Check sheet for the modelled part. Datum: model origin and axes. Units: mm. A direction names the side the tool comes from. Coordinates: 2 decimals unless noted, no trailing zeros. Write each loop counter-clockwise with the first axis right and the second up, starting at its lowest first coordinate (ties: lowest second). Pieces come first, ordered by that corner, then holes. Notation, with made-up numbers: (-31.5, 13.5) - (21.5, 13.5) arc R32 cw to (21.5, 50.5) - close; hole circle Ø9 at (18.25, 72.25). An arc over 180 degrees is marked (long way). Use one line per item in the form item = value. Start each with the question number.
1. Tool access check on faces 1 (the face through (-10, -10, 5)), 2 (the face through (34.997, -21, 15)). Record the directions out of +Z, -Z, +X, -X, +Y, -Y that give a thin tool (end or side, any length) a straight path to the whole face; none if there is none.
2. Cross-section at C-C on y = 8. Record the boundary of the cut face in (x, z), then the cut area to 3 significant figures.
3. Go/stop test with flat-tipped pins: pin 1 Ø1.5 at (x, y) = (-25.5, 10) entering from -Z; pin 2 Ø3.5 at (x, y) = (-15.5, -15.5) entering from +Z; pin 3 Ø5.5 at (x, z) = (30.23, 4.76) entering from +Y; pin 4 Ø1.8 at (x, y) = (15.5, 15.5) entering from -Z. Record where each tip stops, or that it passes through.
4. Scan lines: line 1 along Y through (x, z) = (0, 3); line 2 along X through (y, z) = (6, 15.5); line 3 along Z through (x, y) = (-18.5, 19). Record each from-to range of solid material in increasing order.
5. Cross-section at A-A on x = 0. Record the boundary of the cut face in (y, z), then the cut area to 3 significant figures.
6. Cross-section at D-D on x = 30.5. Record the boundary of the cut face in (y, z), then the cut area to 3 significant figures.
7. Cross-section at B-B on z = 16.5. Record the boundary of the cut face in (x, y), then the cut area to 3 significant figures.
8. Draft check along Z on faces 3 (the face through (-23.86, 1.71, 18.66)), 4 (the face through (30, -19.122, 15)), 5 (the face through (32.385, -20.687, 4.857)), 6 (the face through (-28.084, -20.687, 4.857)). Enter one of: +Z half, -Z half, draft (parallel to the pull), parting line (faces both ways), or undercut.
```python
from build123d import *

# Parameters (mm, degrees)
F0_R     = 1.5
F0_R_2   = 11.253
F1_DEPTH = 5
F3_DEPTH = 25.4
F4_R     = 2.15265
F5_DEPTH = 3.175
F7_DEPTH = 50.943485


with BuildPart() as f1:
    # F0 (on Top) → F1 (new body)
    with BuildSketch(Plane.XY):
        Polygon((25.471742, 21.502992), (-25.471742, 21.502992), (-25.471742, -19.121742), (-34.996742, -19.121742), (-34.996742, -22.296742), (34.996742, -22.296742), (34.996742, -19.121742), (25.471742, -19.121742), align=None)
        with Locations((-15.499994, -15.499994)):
            Circle(F0_R, mode=Mode.SUBTRACT)
        with Locations((15.499994, -15.499994)):
            Circle(F0_R, mode=Mode.SUBTRACT)
        Circle(F0_R_2, mode=Mode.SUBTRACT)
        with Locations((-15.499994, 15.499994)):
            Circle(F0_R, mode=Mode.SUBTRACT)
        with Locations((15.499994, 15.499994)):
            Circle(F0_R, mode=Mode.SUBTRACT)
    extrude(amount=F1_DEPTH)

    # F2 (on face) → F3 (join)
    with BuildSketch(Plane.XY.offset(5)):
        Polygon((-34.996742, -19.121742), (-34.996742, -22.296742), (-22.296742, -22.296742), (-22.296742, 21.502992), (-25.471742, 21.502992), (-25.471742, -19.121742), align=None)
        Polygon((25.471742, -19.121742), (25.471742, 21.502992), (22.296742, 21.502992), (22.296742, -22.296742), (34.996742, -22.296742), (34.996742, -19.121742), align=None)
    extrude(amount=F3_DEPTH)

    # F4 (on face) → F5 (cut, through all)
    with BuildSketch(Plane(origin=(0, -19.121742, 0), x_dir=(-1, 0, 0), z_dir=(0, 1, 0))):
        with Locations((30.234242, 4.7625)):
            Circle(F4_R)
        with Locations((30.234242, 25.6375)):
            Circle(F4_R)
        with Locations((-30.234242, 25.6375)):
            Circle(F4_R)
        with Locations((-30.234242, 4.7625)):
            Circle(F4_R)
    extrude(amount=-F5_DEPTH, mode=Mode.SUBTRACT)

    # F6 (on face) → F7 (cut, through all)
    with BuildSketch(Plane.YZ.offset(25.471742)):
        Polygon((21.502992, 6.5875), (21.502992, 30.4), (-17.534242, 30.4), align=None)
    extrude(amount=-F7_DEPTH, mode=Mode.SUBTRACT)


solid = f1.part
```
Final values:
q1.face_1 = +Z, +Y, -Y
q1.face_2 = +Z, -Z, +X, +Y, -Y
q2.outline = (-25.47, 0) - (-7.91, 0) - (-7.91, 5) - (-22.3, 5) - (-22.3, 14.82) - (-25.47, 14.82) - close; (7.91, 0) - (25.47, 0) - (25.47, 14.82) - (22.3, 14.82) - (22.3, 5) - (7.91, 5) - close
q2.area = 238 mm²
q3.pin_1 = 0
q3.pin_2 = 5
q3.pin_3 = -19.12
q3.pin_4 = through
q4.line_1 = -22.3 to -11.25, 11.25 to 21.5
q4.line_2 = -25.47 to -22.3, 22.3 to 25.47
q4.line_3 = 0 to 5
q5.outline = (-22.3, 0) - (-11.25, 0) - (-11.25, 5) - (-22.3, 5) - close; (11.25, 0) - (21.5, 0) - (21.5, 5) - (11.25, 5) - close
q5.area = 106 mm²
q6.outline = (-22.3, 0) - (-19.12, 0) - (-19.12, 2.63) - (-22.3, 2.63) - close; (-22.3, 6.9) - (-19.12, 6.9) - (-19.12, 23.5) - (-22.3, 23.5) - close; (-22.3, 27.77) - (-19.12, 27.77) - (-19.12, 30.4) - (-22.3, 30.4) - close
q6.area = 69.4 mm²
q7.outline = (-35, -22.3) - (-22.3, -22.3) - (-22.3, 5.25) - (-25.47, 5.25) - (-25.47, -19.12) - (-35, -19.12) - close; (22.3, -22.3) - (35, -22.3) - (35, -19.12) - (25.47, -19.12) - (25.47, 5.25) - (22.3, 5.25) - close
q7.area = 235 mm²
q8.face_3 = +Z half
q8.face_4 = draft
q8.face_5 = undercut
q8.face_6 = undercut
